Check sheet for the modelled part. Datum: model origin and axes. Units: mm. A direction names the side the tool comes from. Round coordinates to 2 decimals unless told otherwise and drop trailing zeros. Write each loop counter-clockwise with the first axis right and the second up, starting at its lowest first coordinate (ties: lowest second). Pieces come first, ordered by that corner, then holes.
from build123d import *

# Parameters (mm, degrees)
F0_W        = 4
F0_H        = 35
F1_DEPTH    = 15
F2_T1_DEPTH = 15
F3_T1_DEPTH = 29.2746233567
F5_DEPTH    = 47
F6_DEPTH    = 5.1
F7_R        = 3
F8_R        = 43.7697785777


# Not quite as in the source:
# - a fillet or chamfer that OpenCascade refuses, or shapes differently, is made with other operations: its cross-section is extruded or revolved along the edge and cut away or added


with BuildPart() as f1:
    # F0 (on Top) → F1 (new body)
    with BuildSketch(Plane.XY):
        with Locations((-2, 17.5)):
            Rectangle(F0_W, F0_H)
        with BuildLine():
            Line((-4, 35), (0, 35))
            ThreePointArc((0, 35), (3.0631994803, 17.6178971132), (2, 0))
            Line((2, 0), (4, 0))
            ThreePointArc((4, 0), (5.0631994803, 17.6178971132), (2, 35))
            ThreePointArc((2, 35), (-1, 38), (-4, 35))
        make_face()
    extrude(amount=F1_DEPTH)

    # F2: fillet of radius 0.3232070394 on 1 edges, made by hand

    # F2_s2 → F2_t1 (join)
    with BuildSketch(Plane.XY):
        with BuildLine():
            ThreePointArc((0, 32.6758460939), (0.2811660755, 32.9963072424), (0.635477172, 32.7592136813))
            ThreePointArc((0.635477172, 32.7592136813), (0.3263947733, 33.8820616974), (0, 35))
            Line((0, 35), (0, 32.6758460939))
        make_face()
    extrude(amount=F2_T1_DEPTH)

    # F3: fillet of radius 2.6852748766 on 1 edges, made by hand

    # F3_s2 → F3_t1 (cut)
    with BuildSketch(Plane.XY.offset(-7.1373116784)):
        with BuildLine():
            ThreePointArc((2.4511484812, 2.8190530195), (2.7567902003, 1.1519659503), (4, 0))
            Line((4, 0), (2, 0))
            ThreePointArc((2, 0), (2.2389229437, 1.4073902438), (2.4511484812, 2.8190530195))
        make_face()
    extrude(amount=F3_T1_DEPTH, mode=Mode.SUBTRACT)

    # F4 (on face) → F5 (cut)
    with BuildSketch(Plane.XZ):
        with BuildLine():
            ThreePointArc((-3.15, 6.5), (-2, 5.35), (-0.85, 6.5))
            Line((-0.85, 6.5), (-2, 6.5))
            Line((-2, 6.5), (-3.15, 6.5))
        make_face()
        with BuildLine():
            ThreePointArc((-0.85, 6.5), (-1.0061251438, 7.0785436631), (-1.4321091654, 7.5))
            ThreePointArc((-1.4321091654, 7.5), (-2, 7.35), (-2.5678908346, 7.5))
            ThreePointArc((-2.5678908346, 7.5), (-2.9938748562, 7.0785436631), (-3.15, 6.5))
            Line((-3.15, 6.5), (-2, 6.5))
            Line((-2, 6.5), (-0.85, 6.5))
        make_face()
        with BuildLine():
            ThreePointArc((-2.5678908346, 7.5), (-2.9938748562, 7.9214563369), (-3.15, 8.5))
            Line((-3.15, 8.5), (-3.15, 6.5))
            ThreePointArc((-3.15, 6.5), (-2.9938748562, 7.0785436631), (-2.5678908346, 7.5))
        make_face()
        with BuildLine():
            Line((-0.85, 6.5), (-0.85, 8.5))
            ThreePointArc((-0.85, 8.5), (-1.0061251438, 7.9214563369), (-1.4321091654, 7.5))
            ThreePointArc((-1.4321091654, 7.5), (-1.0061251438, 7.0785436631), (-0.85, 6.5))
        make_face()
        with BuildLine():
            ThreePointArc((-1.4321091654, 7.5), (-1.0061251438, 7.9214563369), (-0.85, 8.5))
            Line((-0.85, 8.5), (-2, 8.5))
            Line((-2, 8.5), (-3.15, 8.5))
            ThreePointArc((-3.15, 8.5), (-2.9938748562, 7.9214563369), (-2.5678908346, 7.5))
            ThreePointArc((-2.5678908346, 7.5), (-2, 7.35), (-1.4321091654, 7.5))
        make_face()
        with BuildLine():
            Line((-2, 8.5), (-0.85, 8.5))
            ThreePointArc((-0.85, 8.5), (-2, 9.65), (-3.15, 8.5))
            Line((-3.15, 8.5), (-2, 8.5))
        make_face()
    extrude(amount=-F5_DEPTH, mode=Mode.SUBTRACT)

    # F4 (on face) → F6 (join)
    with BuildSketch(Plane.XZ):
        with BuildLine():
            Line((-2, 8.5), (-0.85, 8.5))
            ThreePointArc((-0.85, 8.5), (-2, 9.65), (-3.15, 8.5))
            Line((-3.15, 8.5), (-2, 8.5))
        make_face()
        with BuildLine():
            ThreePointArc((-1.4321091654, 7.5), (-1.0061251438, 7.9214563369), (-0.85, 8.5))
            Line((-0.85, 8.5), (-2, 8.5))
            Line((-2, 8.5), (-3.15, 8.5))
            ThreePointArc((-3.15, 8.5), (-2.9938748562, 7.9214563369), (-2.5678908346, 7.5))
            ThreePointArc((-2.5678908346, 7.5), (-2, 7.35), (-1.4321091654, 7.5))
        make_face()
        with BuildLine():
            ThreePointArc((-3.15, 6.5), (-2, 5.35), (-0.85, 6.5))
            Line((-0.85, 6.5), (-2, 6.5))
            Line((-2, 6.5), (-3.15, 6.5))
        make_face()
        with BuildLine():
            ThreePointArc((-0.85, 6.5), (-1.0061251438, 7.0785436631), (-1.4321091654, 7.5))
            ThreePointArc((-1.4321091654, 7.5), (-2, 7.35), (-2.5678908346, 7.5))
            ThreePointArc((-2.5678908346, 7.5), (-2.9938748562, 7.0785436631), (-3.15, 6.5))
            Line((-3.15, 6.5), (-2, 6.5))
            Line((-2, 6.5), (-0.85, 6.5))
        make_face()
        with BuildLine():
            Line((-0.85, 6.5), (-0.85, 8.5))
            ThreePointArc((-0.85, 8.5), (-1.0061251438, 7.9214563369), (-1.4321091654, 7.5))
            ThreePointArc((-1.4321091654, 7.5), (-1.0061251438, 7.0785436631), (-0.85, 6.5))
        make_face()
        with BuildLine():
            ThreePointArc((-2.5678908346, 7.5), (-2.9938748562, 7.9214563369), (-3.15, 8.5))
            Line((-3.15, 8.5), (-3.15, 6.5))
            ThreePointArc((-3.15, 6.5), (-2.9938748562, 7.0785436631), (-2.5678908346, 7.5))
        make_face()
    extrude(amount=-F6_DEPTH)

    # F7
    f7_edges = [f1.edges().sort_by_distance(p)[0] for p in [
        (0, 0, 7.5),
    ]]
    fillet(f7_edges, radius=F7_R)

    # F8
    f8_edges = [f1.edges().sort_by_distance(p)[0] for p in [
        (2, 35, 7.5),
    ]]
    fillet(f8_edges, radius=F8_R)


solid = f1.part
1. Sectioned sample at C-C, the plane x = -2. Enter the section's corners in (y, z), plus the area to 3 significant figures.
2. Scan lines: line 1 along X through (y, z) = (16.5, 6); line 2 along X through (y, z) = (28, 9.5); line 3 along X through (y, z) = (6, 11.5). Record each from-to range of solid material in increasing order.
3. Go/stop test with flat-tipped pins: pin 1 (3 mm diameter, centred on y = 13, z = 6.5, fed in from +X); pin 2 (4.5 mm diameter, centred on y = 20.5, z = 9, fed in from +X); pin 3 (2 mm diameter, centred on y = 32, z = 10, fed in from +X); pin 4 (2.5 mm diameter, centred on x = -2, z = 8, fed in from +Y). Record where each tip stops, or that it passes through.
4. Sectioned sample at A-A, the plane y = 8. Enter the section's corners in (x, z).
5. Release check for a two-part mould opening along Z. For faces 1 (the flat face through (-0.5, 19.3, 15)), 2 (the flat face through (-3.15, 21, 8)), 3 (the cylindrical face through (3.035, 18.091, 7.395)), 4 (the flat face through (-0.5, 19.3, 0)) record: released by +Z, released by -Z, zero draft, split by the parting line, or undercut.
6. Sectioned sample at B-B, the plane y = 36.5. Enter the section's corners in (x, z), plus the area to 3 significant figures.
7. Set-up check for faces 5 (the cylindrical face through (5.122, 16.41, 7.395)), 6 (the flat face through (-2, 5.1, 8)), 7 (the flat face through (0, 18, 7)): record each of +Z, -Z, +X, -X, +Y, -Y from which the full face is reachable in a straight line by a thin tool's end or side.
Computed values:
1. outline: (0.17, 0) - (37.83, 0) - (37.83, 5.35) - (5.1, 5.35) - (5.1, 9.65) - (37.83, 9.65) - (37.83, 15) - (0.17, 15) - close
1. area: 424 mm2
2. line 1: x = -4 to -3.04, -0.96 to 0, 3.12 to 5.12
2. line 2: x = -4 to -2.57, -1.43 to 0, 1.74 to 3.74
2. line 3: x = -4 to 0, 2.83 to 4.83
3. pin 1: stops at x = 5.19
3. pin 2: stops at x = 5.02
3. pin 3: stops at x = 3.08
3. pin 4: stops at y = 38
4. outline: (-4, 0) - (0, 0) - (0, 15) - (-4, 15) - close; (3, 0) - (5, 0) - (5, 15) - (3, 15) - close; hole (-3.15, 6.5) arc R1.15 ccw to (-0.85, 6.5) - (-0.85, 8.5) arc R1.15 ccw to (-3.15, 8.5) - close
5. face 1: released by +Z
5. face 2: undercut
5. face 3: zero draft
5. face 4: released by -Z
6. outline: (-3.6, 0) - (1.6, 0) - (1.6, 15) - (-3.6, 15) - close; hole (-3.15, 6.5) arc R1.15 ccw to (-0.85, 6.5) - (-0.85, 8.5) arc R1.15 ccw to (-3.15, 8.5) - close
6. area: 69.2 mm2
7. face 5: +Z, -Z, +X
7. face 6: +Y
7. face 7: +Z, -Z, -Y
